Input: part model. Units: mm. Frame: model coordinates. A direction names the side the tool comes from. Coordinates: 2 decimals unless noted, no trailing zeros. Loops run counter-clockwise (first coordinate to the right, second up) from the corner with the lowest first, then second, coordinate; pieces in that order, holes last.
```python
from build123d import *

# Parameters (mm, degrees)
BOSS_EXTRUDE1_DEPTH = 19.05
SKETCH2_W           = 17.018
SKETCH2_H           = 22.225
BOSS_EXTRUDE2_DEPTH = 3.175
SKETCH3_W           = 107.95
SKETCH3_H           = 3.513776003
BOSS_EXTRUDE3_DEPTH = 69.85
FILLET1_R           = 0.508
SKETCH4_R           = 8.54075
CUT_EXTRUDE1_DEPTH  = 26.738776003
SKETCH8_R           = 63.5
CUT_EXTRUDE2_DEPTH  = 26.738776003
SKETCH9_W           = 3.175
SKETCH9_H           = 28.913776003
BOSS_EXTRUDE4_DEPTH = 63.5
SKETCH10_W          = 107.95
SKETCH10_H          = 28.913776003
BOSS_EXTRUDE5_DEPTH = 3.175
SKETCH11_W          = 1.5875
SKETCH11_H          = 7.62
CUT_EXTRUDE3_DEPTH  = 63.5


with BuildPart() as part:
    # Sketch1 → Boss-Extrude1 (new body)
    with BuildSketch(Plane.XY):
        Polygon((8.80657951, 0), (-8.80657951, 0), (-11.98157951, -3.175), (11.98157951, -3.175), align=None)
    extrude(amount=BOSS_EXTRUDE1_DEPTH)

    # Sketch2 → Boss-Extrude2 (add)
    with BuildSketch(Plane(origin=(0, 0, 0), x_dir=(-1, 0, 0), z_dir=(0, 0, -1))):
        with Locations((0, 7.9375)):
            Rectangle(SKETCH2_W, SKETCH2_H)
    extrude(amount=-BOSS_EXTRUDE2_DEPTH)

    # Sketch3 → Boss-Extrude3 (add)
    with BuildSketch(Plane(origin=(0, 0, 0), x_dir=(-1, 0, 0), z_dir=(0, 0, -1))):
        with Locations((0, 20.806888001)):
            Rectangle(SKETCH3_W, SKETCH3_H)
    extrude(amount=-BOSS_EXTRUDE3_DEPTH)

    # Fillet1
    fillet1_edges = [part.edges().sort_by_distance(p)[0] for p in [
        (11.98157951, -3.175, 9.525),
        (-11.98157951, -3.175, 9.525),
    ]]
    fillet(fillet1_edges, radius=FILLET1_R)

    # Sketch4 → Cut-Extrude1 (cut, through all)
    with BuildSketch(Plane(origin=(0, 22.563776003, 0), x_dir=(1, 0, 0), z_dir=(0, 1, 0))):
        with Locations((12.7, -33.9190628)):
            Circle(SKETCH4_R)
        with Locations((-12.7, -33.9190628)):
            Circle(SKETCH4_R)
    extrude(amount=-CUT_EXTRUDE1_DEPTH, mode=Mode.SUBTRACT)

    # Sketch8 → Cut-Extrude2 (cut, through all)
    with BuildSketch(Plane(origin=(0, 22.563776003, 0), x_dir=(1, 0, 0), z_dir=(0, 1, 0))):
        with Locations((0, -127)):
            Circle(SKETCH8_R)
    extrude(amount=-CUT_EXTRUDE2_DEPTH, mode=Mode.SUBTRACT)

    # Sketch9 → Boss-Extrude4 (add)
    with BuildSketch(Plane(origin=(0, 0, 0), x_dir=(-1, 0, 0), z_dir=(0, 0, -1))):
        with Locations((52.3875, 8.106888001)):
            Rectangle(SKETCH9_W, SKETCH9_H)
        with Locations((-52.3875, 8.106888001)):
            Rectangle(SKETCH9_W, SKETCH9_H)
    extrude(amount=-BOSS_EXTRUDE4_DEPTH)

    # Sketch10 → Boss-Extrude5 (add)
    with BuildSketch(Plane(origin=(0, 0, 0), x_dir=(-1, 0, 0), z_dir=(0, 0, -1))):
        with Locations((0, 8.106888001)):
            Rectangle(SKETCH10_W, SKETCH10_H)
    extrude(amount=BOSS_EXTRUDE5_DEPTH)

    # Sketch11 → Cut-Extrude3 (cut)
    with BuildSketch(Plane.XY.offset(63.5)):
        with Locations((51.59375, -2.54)):
            Rectangle(SKETCH11_W, SKETCH11_H)
        with Locations((-51.59375, -2.54)):
            Rectangle(SKETCH11_W, SKETCH11_H)
    extrude(amount=-CUT_EXTRUDE3_DEPTH, mode=Mode.SUBTRACT)


solid = part.part
```
Item 1: Mould query, pull axis Y, two halves, no side actions, for faces 4 (the face through (1, 22.564, 34)), 5 (the face through (0, 0, 12)), 6 (the face through (-52, 9, 63.5)). Classes: +Y half, -Y half, draft (parallel to the pull), parting line (faces both ways), or undercut.
Result:
face 4: +Y half
face 5: undercut
face 6: draft
Item 2: Section query C-C (y = 11.25). Output: boundary loops of the cut face in (x, z) (3 decimals), then the cut area to 3 significant figures.
Result:
outline: (-53.975, -3.175) - (53.975, -3.175) - (53.975, 63.5) - (50.8, 63.5) - (50.8, 0) - (8.509, 0) - (8.509, 3.175) - (-8.509, 3.175) - (-8.509, 0) - (-50.8, 0) - (-50.8, 63.5) - (-53.975, 63.5) - close
area: 800 mm2
Item 3: Section query B-B (x = -12.7). Output: boundary loops of the cut face in (y, z) (3 decimals), then the cut area to 3 significant figures.
Result:
outline: (-6.35, -3.175) - (22.564, -3.175) - (22.564, 25.378) - (19.05, 25.378) - (19.05, 0) - (-6.35, 0) - close; (19.05, 42.46) - (22.564, 42.46) - (22.564, 64.783) - (19.05, 64.783) - close
area: 259 mm2
Item 4: Reachability of faces 1 (the face through (-8.509, 9, 2)), 2 (the face through (52.388, -3, 32)), 3 (the face through (0.4, 20.8, 63.5)) from +Z, -Z, +X, -X, +Y, -Y: full face, straight path, thin tool, end or side. Return the list, or none.
Result:
face 1: +Z
face 2: +Z, -Y
face 3: +Z, +Y, -Y
Item 5: Contact query for flat-ended pins moving along their axis: P1, Ø2.5, axis at x = 53, y = 10, coming from the +Z side; P2, Ø3, axis at x = 21.5, z = 8.5, coming from the -Y side; P3, Ø5, axis at x = -3.5, y = 9.5, coming from the +Z side (3 decimals). Output: stop coordinate, or through.
Result:
P1: stops at z = 63.5
P2: stops at y = 19.05
P3: stops at z = 3.175
Item 6: Line query: L1, parallel to X at y = -1.5, z = 58 (1 decimal); L2, parallel to X at y = 18.75, z = 44 (3 decimals); L3, parallel to Y at x = 5, z = 10 (3 decimals). Output: solid intervals per line, ascending.
Result:
L1: x = -54 to -52.4, 52.4 to 54
L2: x = -53.975 to -50.8, 50.8 to 53.975
L3: y = -3.175 to 0, 19.05 to 22.564
Item 7: Section query A-A (z = 41). Count the separate pieces of the cut face and the enclosed holes in it, then the cut area to 3 significant figures.
Result:
separate pieces: 3
enclosed holes: 0
area: 449 mm2
